Part model, mm, in its own coordinate system. A direction names the side the tool comes from. Round coordinates to 2 decimals unless told otherwise and drop trailing zeros. Write each loop counter-clockwise with the first axis right and the second up, starting at its lowest first coordinate (ties: lowest second). Pieces come first, ordered by that corner, then holes.
```python
from build123d import *

# Parameters (mm, degrees)
F0_W          = 12.0142
F0_H          = 5.7658
F1_DEPTH      = 5.08
F2_W          = 12.0142
F2_H          = 8.509
F3_DEPTH      = 4.2418
F4_R          = 0.762
F6_W          = 4.1768109557
F6_H          = 2.54
F7_DEPTH      = 4.2418
F5_W          = 3.302
F5_H          = 2.54
F8_DEPTH      = 4.318
F8_DEPTH_BACK = 3.048


with BuildPart() as f1:
    # F0 (on Top) → F1 (new body)
    with BuildSketch(Plane.XY):
        Rectangle(F0_W, F0_H)
    extrude(amount=F1_DEPTH)

    # F2 (on Top) → F3 (join)
    with BuildSketch(Plane.XY):
        Rectangle(F2_W, F2_H)
    extrude(amount=-F3_DEPTH)

    # F4
    f4_edges = [f1.edges().sort_by_distance(p)[0] for p in [
        (6.0071, 0, 5.08),
        (0, 2.8829, 5.08),
        (-6.0071, 0, 5.08),
        (0, -2.8829, 5.08),
    ]]
    fillet(f4_edges, radius=F4_R)

    # F6 (on Top) → F7 (cut)
    with BuildSketch(Plane.XY):
        with Locations((-3.4931976115, 0)):
            Rectangle(F6_W, F6_H)
    extrude(amount=-F7_DEPTH, mode=Mode.SUBTRACT)

    # F5 (on Top) → F8 (cut, two sides)
    with BuildSketch(Plane.XY) as f8_sk:
        Rectangle(F5_W, F5_H)
    extrude(amount=-F8_DEPTH, mode=Mode.SUBTRACT)
    extrude(f8_sk.sketch, amount=F8_DEPTH_BACK, mode=Mode.SUBTRACT)


solid = f1.part
```
Q1. Cut at D-D on z = 2.5. Write the cut outline in (x, y), plus the area to 3 significant figures.
Values follow:
outline: (-6.01, -2.88) - (6.01, -2.88) - (6.01, 2.88) - (-6.01, 2.88) - close; hole (-1.65, -1.27) - (1.65, -1.27) - (1.65, 1.27) - (-1.65, 1.27) - close
area: 60.9 mm2
Q2. Cut at C-C on y = -1. Write the cut outline in (x, z), plus the area to 3 significant figures.
Values follow:
outline: (-6.01, -4.24) - (-5.58, -4.24) - (-5.58, 0) - (-1.65, 0) - (-1.65, 3.05) - (1.65, 3.05) - (1.65, -4.24) - (6.01, -4.24) - (6.01, 4.32) arc R0.76 ccw to (5.25, 5.08) - (-5.25, 5.08) arc R0.76 ccw to (-6.01, 4.32) - close
area: 71.0 mm2
Q3. Wall check: L1, parallel to Y at x = 1.5, z = -1.5; L2, parallel to Y at x = 0.25, z = 1; L3, parallel to X at y = 0.75, z = -2. Give the ranges that are in metal, low to high.
Values follow:
L1: y = -4.25 to -1.27, 1.27 to 4.25
L2: y = -2.88 to -1.27, 1.27 to 2.88
L3: x = -6.01 to -5.58, 1.65 to 6.01
Q4. Mould opens along X. For faces 1 (the flat face through (-6.007, 0, 0)), 2 (the flat face through (-1, -1.27, -1)), 3 (the flat face through (6.007, 0, 0)) say: +X half, -X half, draft (parallel to the pull), parting line (faces both ways), or undercut.
Values follow:
face 1: -X half
face 2: undercut
face 3: +X half
Q5. Cut at A-A on z = -1.5. Write the cut outline in (x, y).
Values follow:
outline: (-6.01, -4.25) - (6.01, -4.25) - (6.01, 4.25) - (-6.01, 4.25) - close; hole (-5.58, -1.27) - (1.65, -1.27) - (1.65, 1.27) - (-5.58, 1.27) - close
Q6. Drop flat-ended pins along their axis: pin 1 (3.5 mm diameter, centred on x = 1.5, z = 3, fed in from -Y); pin 2 (2 mm diameter, centred on x = -1, y = 0, fed in from -Z). Give the stop position or say it passes through.
Values follow:
pin 1: stops at y = -2.88
pin 2: stops at z = 0
Q7. Which spindle directions (+Z, -Z, +X, -X, +Y, -Y) get a long thin tool onto all of the face, cutting with end or side? Do faces 4 (the flat face through (0, 0, 3.048)), 5 (the flat face through (0, -4, 0)), 6 (the flat face through (0, 4, 0)), 7 (the flat face through (0, -4.254, -2)). Say none if no direction does.
Values follow:
face 4: -Z
face 5: +Z, +X, -X, -Y
face 6: +Z, +X, -X, +Y
face 7: +Z, -Z, +X, -X, -Y
Q8. Cut at B-B on x = -3.5. Write the cut outline in (y, z), plus the area to 3 significant figures.
Values follow:
outline: (-4.25, -4.24) - (-1.27, -4.24) - (-1.27, 0) - (1.27, 0) - (1.27, -4.24) - (4.25, -4.24) - (4.25, 0) - (2.88, 0) - (2.88, 4.32) arc R0.76 ccw to (2.12, 5.08) - (-2.12, 5.08) arc R0.76 ccw to (-2.88, 4.32) - (-2.88, 0) - (-4.25, 0) - close
area: 54.4 mm2
